Work out the finished part from the listing and answer in its coordinate system (mm). Round coordinates to 2 decimals unless told otherwise and drop trailing zeros. Write each loop counter-clockwise with the first axis right and the second up, starting at its lowest first coordinate (ties: lowest second). Pieces come first, ordered by that corner, then holes. Notation, with made-up numbers: M 30.25,77.25 L 49.25,77.25 A33 cw 49.25,115.25 Z; hole C -35,16 d5. An arc over 180 degrees is marked long. One line per item, written item: value. Start each with the question number.
Q1. Find section B-B (x = -52). Write down the section's boundary in (y, z).
Q2. Find section A-A (z = -11.25). Write down the section's boundary in (x, y).
Q3. The mould has two halves that part along X. Classify faces 1 (the cylindrical face through (1.408, 8.383, -6.439)), 2 (the flat face through (16.424, 6, -6)), 3 (the flat face through (-22, 12.7, -6)): released by +X, released by -X, zero draft, split by the parting line, or undercut.
Q4. Consider probe 1 along X at (y, z) = (5.75, -5.5); probe 2 along X at (y, z) = (7.25, -12); probe 3 along Y at (x, z) = (-45, -8.75). Determine where each line is inside the solid, lowest interval first.
from build123d import *

# Parameters (mm, degrees)
BOSS_EXTRUDE1_DEPTH = 12.7
CUT_EXTRUDE1_DEPTH  = 12.7
BOSS_EXTRUDE3_START = -12.7
SKETCH3_W           = 75
SKETCH3_H           = 12.7
SKETCH3_R           = 2.05
BOSS_EXTRUDE3_DEPTH = 12.7
SKETCH4_R           = 2.05
CUT_EXTRUDE2_DEPTH  = 21.7


with BuildPart() as part:
    # Sketch1 → Boss-Extrude1 (new body)
    with BuildSketch(Plane(origin=(0, 0, 0), x_dir=(1, 0, 0), z_dir=(0, 1, 0))):
        Polygon((-58.57612782, 0), (16.42387218, 0), (16.42387218, 5), (-37.711466165, 5), (-37.711466165, 10), (-58.57612782, 10), align=None)
    extrude(amount=BOSS_EXTRUDE1_DEPTH)

    # Sketch2 → Cut-Extrude1 (cut)
    with BuildSketch(Plane(origin=(0, 0, -10), x_dir=(-1, 0, 0), z_dir=(0, 0, -1))):
        with BuildLine():
            ThreePointArc((41.243796992, 6.35), (43.293796992, 4.3), (45.343796992, 6.35))
            Line((45.343796992, 6.35), (41.243796992, 6.35))
        make_face()
        with BuildLine():
            Line((41.243796992, 6.35), (45.343796992, 6.35))
            ThreePointArc((45.343796992, 6.35), (43.293796992, 8.4), (41.243796992, 6.35))
        make_face()
        with BuildLine():
            ThreePointArc((55.043796992, 6.35), (52.993796992, 8.4), (50.943796992, 6.35))
            Line((50.943796992, 6.35), (55.043796992, 6.35))
        make_face()
        with BuildLine():
            Line((55.043796992, 6.35), (50.943796992, 6.35))
            ThreePointArc((50.943796992, 6.35), (52.993796992, 4.3), (55.043796992, 6.35))
        make_face()
    extrude(amount=-CUT_EXTRUDE1_DEPTH, mode=Mode.SUBTRACT)

    # Sketch3 → Boss-Extrude3 (add)
    with BuildSketch(Plane.XY.offset(BOSS_EXTRUDE3_START)):
        with Locations((-21.07612782, 6.35)):
            Rectangle(SKETCH3_W, SKETCH3_H)
        with Locations(Location((-52.993796992, 6.35, 0), (0, 0, 180))):
            Circle(SKETCH3_R, mode=Mode.SUBTRACT)
        with Locations(Location((-43.293796992, 6.35, 0), (0, 0, 180))):
            Circle(SKETCH3_R, mode=Mode.SUBTRACT)
    extrude(amount=BOSS_EXTRUDE3_DEPTH)

    # Sketch4 → Cut-Extrude2 (cut)
    with BuildSketch(Plane(origin=(0, 0, -12.7), x_dir=(-1, 0, 0), z_dir=(0, 0, -1))):
        with Locations((-10.841541353, 6.35)):
            Circle(SKETCH4_R)
        with Locations((-1.141541353, 6.35)):
            Circle(SKETCH4_R)
    extrude(amount=-CUT_EXTRUDE2_DEPTH, mode=Mode.SUBTRACT)


solid = part.part
The answers:
1. outline: M 0,-12.7 L 4.56,-12.7 L 4.56,0 L 0,0 Z; M 8.14,-12.7 L 12.7,-12.7 L 12.7,0 L 8.14,0 Z
2. outline: M -58.58,0 L 16.42,0 L 16.42,12.7 L -58.58,12.7 Z; hole C -52.99,6.35 d4.1; hole C -43.29,6.35 d4.1; hole C 1.14,6.35 d4.1; hole C 10.84,6.35 d4.1
3. face 1: undercut
3. face 2: released by +X
3. face 3: zero draft
4. probe 1: -58.58 to -54.95, -51.03 to -45.25, -41.33 to -0.82, 3.1 to 8.88, 12.8 to 16.42
4. probe 2: -58.58 to -54.84, -51.15 to -45.14, -41.45 to -0.7, 2.98 to 9, 12.68 to 16.42
4. probe 3: 0 to 5.21, 7.49 to 12.7
